Geometry: final body of the model. Coordinates: model frame, mm. Face numbers are marked on the shaded views. A direction names the side the tool comes from. Coordinates: 2 decimals unless noted, no trailing zeros. Loops run counter-clockwise (first coordinate to the right, second up) from the corner with the lowest first, then second, coordinate; pieces in that order, holes last. Notation, with made-up numbers: (64.5, 76) - (80.5, 76) arc R25 cw to (80.5, 111) - close; hole circle Ø4 at (-3.75, 18.5). An arc over 180 degrees is marked (long way). Return JSON: item names as keys, results as strings.
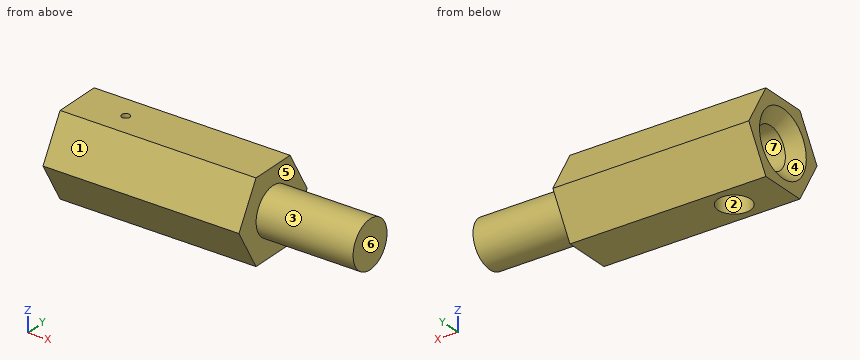
from build123d import *

# Parameters (mm, degrees)
ESTRUSIONE_ESTRUSIONE1_DEPTH        = 12.08
SCHIZZO2_R                          = 1.45
ESTRUSIONE_ESTRUSIONE2_DEPTH        = 5.98
FORO_FILETTATO_M3X0_5_1_D           = 2.5
FORO_FILETTATO_M3X0_5_1_DEPTH       = 8
FORO_FILETTATO_M3X0_5_1_CSINK_D     = 4
FORO_FILETTATO_M3X0_5_1_CSINK_ANGLE = 90
FORO_FILETTATO_M3X0_5_1_TIP         = 0.751075774
TAGLIO_ESTRUSIONE1_REACH            = 20.978
TAGLIO_ESTRUSIONE1_END_RADIUS       = 1.25
SCHIZZO5_R                          = 0.25
TAGLIO_ESTRUSIONE2_REACH            = 20.978
TAGLIO_ESTRUSIONE2_END_RADIUS       = 1.25
SCHIZZO6_R                          = 1


with BuildPart() as part:
    # Schizzo1 → Estrusione-Estrusione1 (new body)
    with BuildSketch(Plane(origin=(0, 0, 0), x_dir=(0, 0, -1), z_dir=(1, 0, 0))):
        Polygon((0, 2.915618859), (-2.525, 1.45780943), (-2.525, -1.45780943), (0, -2.915618859), (2.525, -1.45780943), (2.525, 1.45780943), align=None)
    extrude(amount=ESTRUSIONE_ESTRUSIONE1_DEPTH)

    # Schizzo2 → Estrusione-Estrusione2 (add)
    with BuildSketch(Plane(origin=(12.08, 0, 0), x_dir=(0, 0, -1), z_dir=(1, 0, 0))):
        Circle(SCHIZZO2_R)
    extrude(amount=ESTRUSIONE_ESTRUSIONE2_DEPTH)

    # Foro filettato M3x0.5-1
    with Locations(Plane.ZY):
        with Locations((0, 0)):
            CounterSinkHole(FORO_FILETTATO_M3X0_5_1_D / 2, FORO_FILETTATO_M3X0_5_1_CSINK_D / 2, depth=FORO_FILETTATO_M3X0_5_1_DEPTH, counter_sink_angle=FORO_FILETTATO_M3X0_5_1_CSINK_ANGLE)
            with Locations((0, 0, -(FORO_FILETTATO_M3X0_5_1_DEPTH + FORO_FILETTATO_M3X0_5_1_TIP / 2))):  # 118° drill point
                Cone(0, FORO_FILETTATO_M3X0_5_1_D / 2, FORO_FILETTATO_M3X0_5_1_TIP, mode=Mode.SUBTRACT)

    # Taglio-Estrusione1: up to this cylinder (the profile starts outside it)
    taglio_estrusione1_end = Plane(origin=(3, 0, 0), z_dir=(-1, 0, 0)) * Cylinder(TAGLIO_ESTRUSIONE1_END_RADIUS, 45.456, mode=Mode.PRIVATE)
    # Schizzo5 → Taglio-Estrusione1 (cut, up to the surface)
    with BuildSketch(Plane.XY.offset(2.525), mode=Mode.PRIVATE) as taglio_estrusione1_sk1:
        with Locations((3, 0)):
            Circle(SCHIZZO5_R)
    taglio_estrusione1_tool1 = extrude(taglio_estrusione1_sk1.sketch, amount=-TAGLIO_ESTRUSIONE1_REACH, mode=Mode.PRIVATE) - taglio_estrusione1_end
    add(taglio_estrusione1_tool1.solids().sort_by_distance((3, 0, 2.525))[0], mode=Mode.SUBTRACT)

    # Taglio-Estrusione2: up to this cylinder (the profile starts outside it)
    taglio_estrusione2_end = Plane(origin=(3, 0, 0), z_dir=(-1, 0, 0)) * Cylinder(TAGLIO_ESTRUSIONE2_END_RADIUS, 45.456, mode=Mode.PRIVATE)
    # Schizzo6 → Taglio-Estrusione2 (cut, up to the surface)
    with BuildSketch(Plane(origin=(0, 0, -2.525), x_dir=(-1, 0, 0), z_dir=(0, 0, -1)), mode=Mode.PRIVATE) as taglio_estrusione2_sk1:
        with Locations(Location((-3, 0, 0), (0, 0, 90))):
            Circle(SCHIZZO6_R)
    taglio_estrusione2_tool1 = extrude(taglio_estrusione2_sk1.sketch, amount=-TAGLIO_ESTRUSIONE2_REACH, mode=Mode.PRIVATE) - taglio_estrusione2_end
    add(taglio_estrusione2_tool1.solids().sort_by_distance((3, 0, -2.525))[0], mode=Mode.SUBTRACT)


solid = part.part
Item 1: Section query D-D, the plane y = 2.2. Return loops of the section in (x, z), and give its area (3 significant figures).
Worked out:
{"outline": "(0, -1.24) - (12.08, -1.24) - (12.08, 1.24) - (0, 1.24) - close", "area": "29.9 mm^2"}
Item 2: Section query C-C, the plane x = 10.25. Return loops of the section in (y, z) (3 decimals).
Worked out:
{"outline": "(-2.916, 0) - (-1.458, -2.525) - (1.458, -2.525) - (2.916, 0) - (1.458, 2.525) - (-1.458, 2.525) - close"}
Item 3: Section query A-A, the plane x = 3. Return loops of the section in (y, z) (3 decimals).
Worked out:
{"outline": "(-2.916, 0) - (-1.458, -2.525) - (-1, -2.525) - (-1, -0.75) arc R1.25 cw to (-0.25, 1.225) - (-0.25, 2.525) - (-1.458, 2.525) - close; (0.25, 1.225) arc R1.25 cw to (1, -0.75) - (1, -2.525) - (1.458, -2.525) - (2.916, 0) - (1.458, 2.525) - (0.25, 2.525) - close"}
Item 4: Ray query, probe 1 along Z at (x, y) = (5.25, 0) (3 decimals); probe 2 along Z at (x, y) = (3.25, 0.25) (3 decimals); probe 3 along Y at (x, z) = (3, -1.2). Return the intervals inside material, ascending. Write a range as from..to.
Worked out:
{"probe 1": "-2.525..-1.25, 1.25..2.525", "probe 2": "1.225..2.525", "probe 3": "-2.22..-1, 1..2.22"}
Item 5: Section query B-B, the plane z = -2.2. Return loops of the section in (x, y).
Worked out:
{"outline": "(0, -1.65) - (12.08, -1.65) - (12.08, 1.65) - (0, 1.65) - close; hole circle Ø2 at (3, 0)"}
Item 6: Mould query, pull axis Z, two halves, no side actions, for the marked faces 1, 2, 3 and 4. Classes: +Z half, -Z half, draft (parallel to the pull), parting line (faces both ways), or undercut.
Worked out:
{"face 1": "+Z half", "face 2": "draft", "face 3": "parting line", "face 4": "undercut"}
Item 7: Reachability of the marked faces 5, 6 and 7 from +Z, -Z, +X, -X, +Y, -Y: full face, straight path, thin tool, end or side. Return the list, or none.
Worked out:
{"face 5": "+X", "face 6": "+Z, -Z, +X, +Y, -Y", "face 7": "-X"}
Item 8: First-contact query: pin 1 Ø3 at (x, z) = (7.5, 1) entering from +Y; pin 2 Ø2 at (x, z) = (3.5, 0.5) entering from -Y. Flat tips, straight axial feed; report the tip coordinate or a pass-through.
Worked out:
{"pin 1": "y = 2.92", "pin 2": "y = -2.92"}
